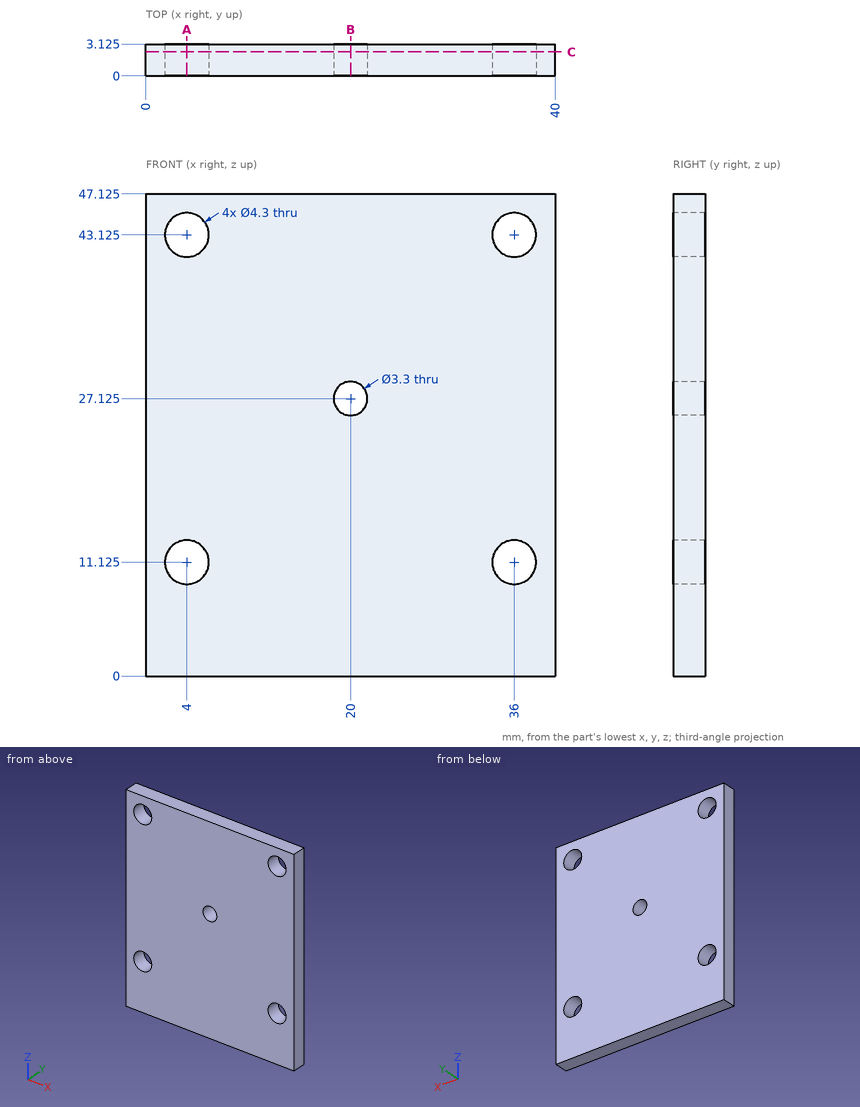
Geometry check sheet. Reference: drawing and pictorial views, mm from the part's lowest x, y, z. Give positions to 0.01 mm unless a question says otherwise; leave off trailing zeros. Loops run counter-clockwise (first coordinate to the right, second up) from the corner with the lowest first, then second, coordinate; pieces in that order, holes last. Notation, with made-up numbers: (-3.5, -38.75) - (44.5, -38.75) arc R14 ccw to (44.5, -31.75) - close; hole circle Ø8 at (16.25, -38). An arc over 180 degrees is marked (long way). Use CSV: the item, a comma, the result in double quotes. Start each with the question number.
Q1. Section check B-B, the plane x = 20. Record the cut outline in (y, z) (3 decimals).
Q2. Section check A-A, the plane x = 4. Record the cut outline in (y, z) (3 decimals), and give its area (3 significant figures).
Q3. Scan lines: probe 1 along Z at (x, y) = (4, 0.8) (3 decimals); probe 2 along Z at (x, y) = (20, 1.9) (3 decimals); probe 3 along X at (y, z) = (0.85, 42). Record each from-to range of solid material in increasing order. Write a range as from..to.
Q4. Section check C-C, the plane y = 2.35. Record the cut outline in (x, z) (3 decimals).
Findings below:
1,outline,"(0, 0) - (3.125, 0) - (3.125, 25.475) - (0, 25.475) - close; (0, 28.775) - (3.125, 28.775) - (3.125, 47.125) - (0, 47.125) - close"
2,outline,"(0, 0) - (3.125, 0) - (3.125, 8.975) - (0, 8.975) - close; (0, 13.275) - (3.125, 13.275) - (3.125, 40.975) - (0, 40.975) - close; (0, 45.275) - (3.125, 45.275) - (3.125, 47.125) - (0, 47.125) - close"
2,area,"120 mm^2"
3,probe 1,"z = 0..8.975, 13.275..40.975, 45.275..47.125"
3,probe 2,"z = 0..25.475, 28.775..47.125"
3,probe 3,"x = 0..2.17, 5.83..34.17, 37.83..40"
4,outline,"(0, 0) - (40, 0) - (40, 47.125) - (0, 47.125) - close; hole circle Ø4.3 at (4, 11.125); hole circle Ø4.3 at (4, 43.125); hole circle Ø3.3 at (20, 27.125); hole circle Ø4.3 at (36, 11.125); hole circle Ø4.3 at (36, 43.125)"
